Work out the finished part from the listing and answer in its coordinate system (mm). Face numbers are marked on the shaded views. Give positions to 0.01 mm unless a question says otherwise; leave off trailing zeros. Loops run counter-clockwise (first coordinate to the right, second up) from the corner with the lowest first, then second, coordinate; pieces in that order, holes last. Notation, with made-up numbers: M 50.5,-31 L 86.5,-31 A6 cw 86.5,-26 Z; hole C -36.5,44 d6. An arc over 180 degrees is marked long. Answer as a JSON object with one key per item and string values. Group by question number.
```python
from build123d import *

# Parameters (mm, degrees)
SCHIZZO1_R                   = 3.5
ESTRUSIONE_ESTRUSIONE1_DEPTH = 5
SCHIZZO3_W                   = 100
SCHIZZO3_H                   = 38
SCHIZZO3_R                   = 4
ESTRUSIONE_ESTRUSIONE2_DEPTH = 5
RACCORDO1_R                  = 5
RACCORDO2_R                  = 7


with BuildPart() as part:
    # Schizzo1 → Estrusione-Estrusione1 (new body)
    with BuildSketch(Plane.XY):
        with BuildLine():
            Line((66, 80), (100, 80))
            Line((100, 80), (100, 0))
            Line((100, 0), (0, 0))
            Line((0, 0), (0, 80))
            Line((0, 80), (34, 80))
            ThreePointArc((34, 80), (50, 64), (66, 80))
        make_face()
        with Locations((31, 61)):
            Circle(SCHIZZO1_R, mode=Mode.SUBTRACT)
        with Locations((69, 61)):
            Circle(SCHIZZO1_R, mode=Mode.SUBTRACT)
    extrude(amount=ESTRUSIONE_ESTRUSIONE1_DEPTH)

    # Schizzo3 → Estrusione-Estrusione2 (add)
    with BuildSketch(Plane(origin=(0, 0, 0), x_dir=(1, 0, 0), z_dir=(0, 1, 0))):
        with Locations((50, -19)):
            Rectangle(SCHIZZO3_W, SCHIZZO3_H)
        with Locations((15, -22.1)):
            Circle(SCHIZZO3_R, mode=Mode.SUBTRACT)
        with Locations((85, -22.1)):
            Circle(SCHIZZO3_R, mode=Mode.SUBTRACT)
    extrude(amount=ESTRUSIONE_ESTRUSIONE2_DEPTH)

    # Raccordo1
    raccordo1_edges = [part.edges().sort_by_distance(p)[0] for p in [
        (50, 5, 5),
    ]]
    fillet(raccordo1_edges, radius=RACCORDO1_R)

    # Raccordo2
    raccordo2_edges = [part.edges().sort_by_distance(p)[0] for p in [
        (50, 0, 0),
    ]]
    fillet(raccordo2_edges, radius=RACCORDO2_R)


solid = part.part
```
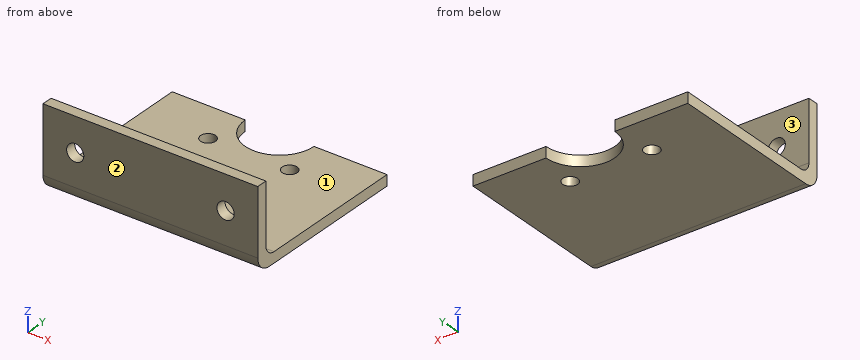
Item 1: A cutting plane is placed at D-D (z = 3.5). Determine the outline of the cut face in (x, y).
Item 2: Given pin 1 Ø4 at (x, z) = (55, 27) entering from +Y; pin 2 Ø12 at (x, y) = (31, 33.5) entering from +Z; pin 3 Ø6 at (y, z) = (56, 6.5) entering from -X; pin 4 Ø3 at (x, z) = (48, 4) entering from -Y, each flat-ended and moving along its own axis, determine where each tip first touches the part or whether it passes through.
Item 3: For a pull along Y with two mould halves and no side action, classify the marked faces 1, 2 and 3 as pulls with the +Y half, pulls with the -Y half, needs draft (parallel to the pull), parting line crosses it, or undercut.
Item 4: A cutting plane is placed at C-C (y = 72). Determine the outline of the cut face in (x, z).
Item 5: Find the intervals of material crossed by probe 1 along X at (y, z) = (2.4, 22.1); probe 2 along Z at (x, y) = (81, 46), in increasing order. Write a range as [from, to].
Item 6: A cutting plane is placed at B-B (z = 22.1). Determine the outline of the cut face in (x, y).
Item 7: A cutting plane is placed at A-A (x = 15). Determine the outline of the cut face in (y, z).
The answers:
{
 "1": {"outline": "M 0,0.94 L 100,0.94 L 100,80 L 66,80 A16 cw 34,80 L 0,80 Z; hole C 31,61 d7; hole C 69,61 d7"},
 "2": {"pin 1": "stops at y = 5", "pin 2": "stops at z = 5", "pin 3": "stops at x = 0", "pin 4": "stops at y = 0.16"},
 "3": {"face 1": "needs draft", "face 2": "pulls with the -Y half", "face 3": "pulls with the +Y half"},
 "4": {"outline": "M 0,0 L 36.14,0 L 36.14,5 L 0,5 Z; M 63.86,0 L 100,0 L 100,5 L 63.86,5 Z"},
 "5": {"probe 1": "x = [0, 11], [19, 81], [89, 100]", "probe 2": "z = [0, 5]"},
 "6": {"outline": "M 0,0 L 11,0 L 11,5 L 0,5 Z; M 19,0 L 81,0 L 81,5 L 19,5 Z; M 89,0 L 100,0 L 100,5 L 89,5 Z"},
 "7": {"outline": "M 0,7 A7 ccw 7,0 L 80,0 L 80,5 L 10,5 A5 cw 5,10 L 5,18.1 L 0,18.1 Z; M 0,26.1 L 5,26.1 L 5,38 L 0,38 Z"}
}
